The listing builds one solid part. Answer for the finished solid, in the listing's coordinates (mm). A direction names the side the tool comes from. Give positions to 0.01 mm unless a question says otherwise; leave off trailing zeros. Order: outer loops, then holes, each group sorted by start corner. A loop starts at its lowest first (then second) coordinate and runs counter-clockwise, first axis right, second up. Notation, with made-up numbers: (12.5, -5) - (18.5, -5) arc R22 ccw to (18.5, 15) - close; hole circle Ø11 at (34.25, 41.5). An arc over 180 degrees is marked (long way). Answer in a Markdown table with one row per item.
from build123d import *

# Parameters (mm, degrees)
F0_R     = 12.827
F1_DEPTH = 2.54
F2_R     = 8.89
F3_DEPTH = 0.635
F5_R     = 25.4
F7_R     = 3.81
F8_DEPTH = 5


# Not quite as in the source:
# - a fillet or chamfer that OpenCascade refuses, or shapes differently, is made with other operations: its cross-section is extruded or revolved along the edge and cut away or added


with BuildPart() as f1:
    # F0 (on Top) → F1 (new body)
    with BuildSketch(Plane.XY):
        Circle(F0_R)
    extrude(amount=-F1_DEPTH)

    # F2 (on face) → F3 (cut)
    with BuildSketch(Plane(origin=(0, 0, -2.54), x_dir=(1, 0, 0), z_dir=(0, 0, -1))):
        Circle(F2_R)
    extrude(amount=-F3_DEPTH, mode=Mode.SUBTRACT)

    # F4: fillet of radius 60.96 on 1 edges, made by hand

    # F4_s1 → F4_t2 (revolve)
    with BuildSketch(Plane.XZ):
        with BuildLine():
            ThreePointArc((8.89, -2.54), (4.5135344509, -2.0639572458), (0.1141253997, -1.905))
            Line((0.1141253997, -1.905), (8.89, -1.905))
            Line((8.89, -1.905), (8.89, -2.54))
        make_face()
    revolve(axis=Axis((0, 0, -1.905), (0, 0, -1)))

    # F5
    f5_edges = [f1.edges().sort_by_distance(p)[0] for p in [
        (-8.89, 0, -2.54),
    ]]
    fillet(f5_edges, radius=F5_R)

    # F6: fillet of radius 2.54 on 1 edges, made by hand

    # F6_s1 → F6_t2 (revolve, cut)
    with BuildSketch(Plane.XZ):
        with BuildLine():
            ThreePointArc((10.2547372433, -2.5384738057), (12.0719517601, -1.8053490766), (12.8274, 0.0026991598))
            Line((12.8274, 0.0026991598), (13.0815365685, 0.0026991598))
            ThreePointArc((13.0815365685, 0.0026991598), (13.0811365685, -1.2686504201), (13.0811365685, -2.54))
            Line((13.0811365685, -2.54), (12.827, -2.7941365685))
            ThreePointArc((12.827, -2.7941365685), (10.5675446967, -2.7941365685), (10.2516075362, -2.7925911022))
            Line((10.2516075362, -2.7925911022), (10.2547372433, -2.5384738057))
        make_face()
    revolve(axis=Axis((0, 0, -2.54), (0, 0, 1)), mode=Mode.SUBTRACT)

    # F7 (on face) → F8 (join)
    with BuildSketch(Plane.XY):
        Circle(F7_R)
    extrude(amount=F8_DEPTH)


solid = f1.part
Item 1: Each of these flat-tipped pins is pushed along its axis until it touches: P1, Ø3, axis at x = 2.5, y = 7, coming from the +Z side; P2, Ø1.5, axis at y = -4.5, z = -1.5, coming from the -X side; P3, Ø10, axis at x = -1, y = 5, coming from the -Z side. Where does it stop, or does it pass through?
Answer block:
| item | result |
|---|---|
| P1 | z = 0 |
| P2 | x = -12 |
| P3 | z = -2.54 |
Item 2: Find section B-B on z = -0.5. Write down the section's boundary in (x, y).
Answer block:
| item | result |
|---|---|
| outline | circle Ø25.55 at (0, 0) |
Item 3: Find section A-A on z = 3. Write down the section's boundary in (x, y), then the cut area to 3 significant figures.
Answer block:
| item | result |
|---|---|
| outline | circle Ø7.62 at (0, 0) |
| area | 45.6 mm² |
Item 4: Consider line 1 (Z direction, x = -0.25, y = -10); line 2 (X direction, y = 9.5, z = -1); line 3 (X direction, y = 9, z = -1.25). Determine where each line is inside the solid, lowest interval first.
Answer block:
| item | result |
|---|---|
| line 1 | -2.53 to 0 |
| line 2 | -8.31 to 8.31 |
| line 3 | -8.67 to 8.67 |
Item 5: Which of the six approach directions +Z, -Z, +X, -X, +Y, -Y give full straight-line access (tool end or side, diameter ignored) to faces 1 (the face through (0, 0, 5)), 2 (the face through (-0.83, -3.72, 2.46))?
Answer block:
| item | result |
|---|---|
| face 1 | +Z, +X, -X, +Y, -Y |
| face 2 | +Z |
